Geometry: final body of the model. Coordinates: model frame, mm. Round coordinates to 2 decimals unless told otherwise and drop trailing zeros. Loops run counter-clockwise (first coordinate to the right, second up) from the corner with the lowest first, then second, coordinate; pieces in that order, holes last. Notation, with made-up numbers: (77, 14.5) - (127, 14.5) arc R25 ccw to (127, 47.5) - close; hole circle Ø7 at (-16.75, -23). An arc over 180 degrees is marked (long way). Answer in a Markdown table with one row per item. Add a question column.
from build123d import *

# Parameters (mm, degrees)
F0_R     = 38.1
F0_R_2   = 12.7
F1_DEPTH = 25.4
F3_DEPTH = 25.4


with BuildPart() as f1:
    # F0 (on Front) → F1 (new body)
    with BuildSketch(Plane.XZ):
        Circle(F0_R)
        Circle(F0_R_2, mode=Mode.SUBTRACT)
    extrude(amount=F1_DEPTH)

    # F2 (on face) → F3 (cut)
    with BuildSketch(Plane.XZ.offset(25.4)):
        with BuildLine():
            ThreePointArc((12.522369, 35.983333), (12.655514, 37.037946), (12.7, 38.1))
            ThreePointArc((12.7, 38.1), (-1.062054, 50.755514), (-12.522369, 35.983333))
            ThreePointArc((-12.522369, 35.983333), (0, 38.1), (12.522369, 35.983333))
        make_face()
        with BuildLine():
            ThreePointArc((-20.295568, -19.05), (-25.748045, -8.62103), (-37.423665, -7.146977))
            ThreePointArc((-37.423665, -7.146977), (-32.995568, -19.05), (-24.901296, -28.836356))
            ThreePointArc((-24.901296, -28.836356), (-21.504544, -24.457992), (-20.295568, -19.05))
        make_face()
        with BuildLine():
            ThreePointArc((24.901296, -28.836356), (32.995568, -19.05), (37.423665, -7.146977))
            ThreePointArc((37.423665, -7.146977), (21.997045, -12.7), (24.901296, -28.836356))
        make_face()
        with BuildLine():
            ThreePointArc((12.522369, 35.983333), (0, 38.1), (-12.522369, 35.983333))
            ThreePointArc((-12.522369, 35.983333), (0, 25.4), (12.522369, 35.983333))
        make_face()
        with BuildLine():
            ThreePointArc((45.695568, -19.05), (43.424538, -11.802478), (37.423665, -7.146977))
            ThreePointArc((37.423665, -7.146977), (32.995568, -19.05), (24.901296, -28.836356))
            ThreePointArc((24.901296, -28.836356), (38.40356, -30.541024), (45.695568, -19.05))
        make_face()
        with BuildLine():
            ThreePointArc((-24.901296, -28.836356), (-32.995568, -19.05), (-37.423665, -7.146977))
            ThreePointArc((-37.423665, -7.146977), (-43.994091, -25.4), (-24.901296, -28.836356))
        make_face()
    extrude(amount=-F3_DEPTH, mode=Mode.SUBTRACT)


solid = f1.part
1) Pull-direction query (X, two-part tool) for faces 1 (the cylindrical face through (-2.75, -12.52, -12.4)), 2 (the cylindrical face through (-32.804, -12.522, 19.378)), 3 (the cylindrical face through (22.12, -12.88, -12.49)), 4 (the cylindrical face through (-0.38, -12.52, -38.1)); classes: pulls with the +X half, pulls with the -X half, needs draft (parallel to the pull), parting line crosses it, or undercut.
2) Section C-C, the plane z = 22. Return the cut outline in (x, y), and give its area (3 significant figures).
3) Section A-A, the plane x = 0. Return the cut outline in (y, z), and give its area (3 significant figures).
4) Section D-D, the plane x = -33. Return the cut outline in (y, z), and give its area (3 significant figures).
5) Contact query for flat-ended pins moving along their axis: pin 1 Ø23 at (x, z) = (0, 0) entering from +Y; pin 2 Ø6 at (y, z) = (-8, -8.5) entering from +X; pin 3 Ø8 at (y, z) = (-8.5, -14) entering from +X; pin 4 Ø2 at (x, y) = (23.5, -12.5) entering from +Z. Output: stop coordinate, or through.
6) Material intervals for line 1 along Z through (x, y) = (0, -18.5); line 2 along X through (y, z) = (-19.5, -0.5); line 3 along Z through (x, y) = (-3, -20.5), sorted ascending. Write a range as from..to.
7) Section B-B, the plane z = 0. Return the cut outline in (x, y), and give its area (3 significant figures).
Evaluation:
| question | item | result |
|---|---|---|
| 1 | face 1 | undercut |
| 1 | face 2 | pulls with the -X half |
| 1 | face 3 | undercut |
| 1 | face 4 | parting line crosses it |
| 2 | outline | (-31.11, -25.4) - (31.11, -25.4) - (31.11, 0) - (-31.11, 0) - close |
| 2 | area | 1,580 mm² |
| 3 | outline | (-25.4, -38.1) - (0, -38.1) - (0, -12.7) - (-25.4, -12.7) - close; (-25.4, 12.7) - (0, 12.7) - (0, 25.4) - (-25.4, 25.4) - close |
| 3 | area | 968 mm² |
| 4 | outline | (-25.4, -6.35) - (0, -6.35) - (0, 19.04) - (-25.4, 19.04) - close |
| 4 | area | 645 mm² |
| 5 | pin 1 | passes through |
| 5 | pin 2 | stops at x = 37.7 |
| 5 | pin 3 | stops at x = 24.09 |
| 5 | pin 4 | stops at z = 30.75 |
| 6 | line 1 | z = -38.1..-12.7, 12.7..25.4 |
| 6 | line 2 | x = -38.1..-12.69, 12.69..38.1 |
| 6 | line 3 | z = -37.98..-12.34, 12.34..25.76 |
| 7 | outline | (-38.1, -25.4) - (-12.7, -25.4) - (-12.7, 0) - (-38.1, 0) - close; (12.7, -25.4) - (38.1, -25.4) - (38.1, 0) - (12.7, 0) - close |
| 7 | area | 1,290 mm² |
